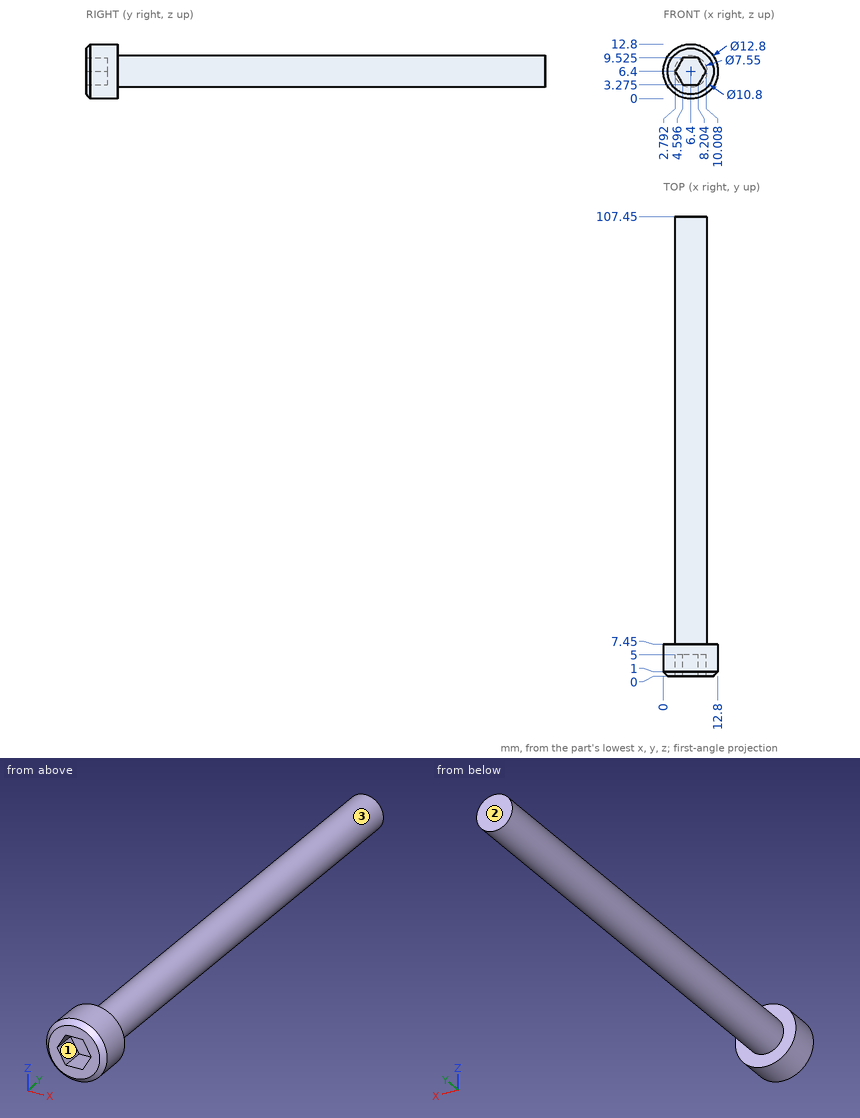
Geometry: see drawing. Coordinates: mm, zero at the bounding-box minimum. Round coordinates to 2 decimals unless told otherwise and drop trailing zeros. Answer as a JSON object with one key per item and string values. Group by question number.
(1) Ray query, line 1 (Y direction, x = 5.75, z = 1.25); line 2 (Y direction, x = 4.75, z = 6); line 3 (Z direction, x = 4.25, y = 91) (1 decimal). Return the intervals inside material, ascending. Write a range as [from, to].
(2) First-contact query: pin 1 (3 mm diameter, centred on x = 6, z = 5.5, fed in from -Y); pin 2 (3 mm diameter, centred on x = 10.5, y = 14.5, fed in from +Z); pin 3 (5 mm diameter, centred on x = 5.5, y = 91, fed in from +Z) (3 decimals). Flat tips, straight axial feed; report the tip coordinate or a pass-through.
(3) Mould query, pull axis Z, two halves, no side actions, for the marked faces 1, 2 and 3. Classes: +Z half, -Z half, draft (parallel to the pull), parting line (faces both ways), or undercut.
Computed values:
{
 "1": {"line 1": "[0, 7.45]", "line 2": "[5, 107.45]", "line 3": "[3.3, 9.5]"},
 "2": {"pin 1": "y = 5", "pin 2": "z = 9.14", "pin 3": "z = 10.175"},
 "3": {"face 1": "undercut", "face 2": "draft", "face 3": "parting line"}
}
